```python
from build123d import *

# Parameters (mm, degrees)
SKETCH2_R           = 3.5
BOSS_EXTRUDE1_DEPTH = 1.2
SKETCH3_R           = 0.875
CUT_EXTRUDE1_DEPTH  = 47.574778582
SKETCH10_R          = 2
CUT_EXTRUDE4_DEPTH  = 33.9
SKETCH6_OUTSIDE_W   = 38.142
SKETCH6_OUTSIDE_H   = 38.142
CUT_EXTRUDE2_DEPTH  = 3
FILLET1_R           = 0.2
BOSS_EXTRUDE2_START = 1.5
SKETCH7_W           = 20
SKETCH7_H           = 16
BOSS_EXTRUDE2_DEPTH = 11.5
CHAMFER2_SIZE       = 0.5
SKETCH8_R           = 0.2
CUT_EXTRUDE3_DEPTH  = 67.283482105
SKETCH9_W           = 1.6
SKETCH9_H           = 1.6


with BuildPart() as part:
    # Sketch1 → Revolve1 (revolve)
    with BuildSketch(Plane.XY):
        Polygon((0, 0), (-8, 0), (-8, -3.7), (-6, -3.7), (-6, -9.7), (-8, -9.7), (-8, -12.7), (-4, -12.7), (-4, -14.2), (-8, -14.2), (-8, -15.2), (-4, -15.2), (-4, -16.7), (-11, -16.7), (-11, -17.7), (-3, -17.7), (-3, -19.2), (-11, -19.2), (-11, -20.2), (-3, -20.2), (-3, -21.7), (-11, -21.7), (-11, -22.7), (-3, -22.7), (-3, -24.2), (-11, -24.2), (-11, -25.2), (-3, -25.2), (-3, -26.7), (-11, -26.7), (-11, -27.7), (-3, -27.7), (-3, -29.2), (-11, -29.2), (-11, -30.2), (-3, -30.2), (-3, -31.7), (-11, -31.7), (-11, -32.7), (-3, -32.7), (-3, -34.2), (-11, -34.2), (-11, -35.2), (-3, -35.2), (-3, -36.7), (-11, -36.7), (-11, -37.7), (-3, -37.7), (-3, -39.2), (-11, -39.2), (-11, -40.2), (-3, -40.2), (-3, -41.7), (-11, -41.7), (-11, -42.7), (0, -42.7), align=None)
    revolve(axis=Axis((0, 0, 0), (0, -1, 0)))

    # Sketch2 → Boss-Extrude1 (add)
    with BuildSketch(Plane(origin=(0, 0, 0), x_dir=(1, 0, 0), z_dir=(0, 1, 0))):
        with Locations(Location((0, 0, 0), (0, 0, 180))):
            Circle(SKETCH2_R)
    extrude(amount=BOSS_EXTRUDE1_DEPTH)

    # Sketch3 → Cut-Extrude1 (cut, through all)
    with BuildSketch(Plane(origin=(0, 1.2, 0), x_dir=(1, 0, 0), z_dir=(0, 1, 0))):
        with Locations(Location((0, 0, 0), (0, 0, 180))):
            Circle(SKETCH3_R)
    extrude(amount=-CUT_EXTRUDE1_DEPTH, mode=Mode.SUBTRACT)

    # Sketch10 → Cut-Extrude4 (cut)
    with BuildSketch(Plane(origin=(0, 1.2, 0), x_dir=(1, 0, 0), z_dir=(0, 1, 0))):
        with Locations(Location((0, 0, 0), (0, 0, 180))):
            Circle(SKETCH10_R)
    extrude(amount=-CUT_EXTRUDE4_DEPTH, mode=Mode.SUBTRACT)

    # Sketch5 → Revolve2 (revolve)
    with BuildSketch(Plane.XY, mode=Mode.PRIVATE) as revolve2_sk:
        Polygon((0, -42.7), (-2.5, -42.7), (-2.5, -57.3), (-5, -57.3), (-5, -60.3), (-1.715415076, -60.3), (-0.315, -62.3), (0, -62.3), align=None)
    revolve(revolve2_sk.sketch.rotate(Axis((0, -62.3, 0), (0, 1, 0)), 270), axis=Axis((0, -62.3, 0), (0, 1, 0)))

    # Sketch6 outside → Cut-Extrude2 (cut)
    with BuildSketch(Plane.XZ.offset(60.3)):
        Rectangle(SKETCH6_OUTSIDE_W, SKETCH6_OUTSIDE_H)
        Polygon((2.020725942, 3.5), (-2.020725942, 3.5), (-4.041451884, 0), (-2.020725942, -3.5), (2.020725942, -3.5), (4.041451884, 0), align=None, mode=Mode.SUBTRACT)
    extrude(amount=-CUT_EXTRUDE2_DEPTH, mode=Mode.SUBTRACT)

    # Fillet1
    fillet1_edges = [part.edges().sort_by_distance(p)[0] for p in [
        (2.020725942, -58.8, 3.5),
        (-2.020725942, -58.8, 3.5),
        (-4.041451884, -58.8, 0),
        (-2.020725942, -58.8, -3.5),
        (2.020725942, -58.8, -3.5),
        (4.041451884, -58.8, 0),
    ]]
    fillet(fillet1_edges, radius=FILLET1_R)

    # Sketch7 → Boss-Extrude2 (add)
    with BuildSketch(Plane(origin=(0, -57.3, 0), x_dir=(1, 0, 0), z_dir=(0, 1, 0)).offset(BOSS_EXTRUDE2_START)):
        with Locations((-5.5, 0)):
            Rectangle(SKETCH7_W, SKETCH7_H)
    extrude(amount=BOSS_EXTRUDE2_DEPTH)

    # Chamfer2
    chamfer2_edges = [part.edges().sort_by_distance(p)[0] for p in [
        (4.5, -55.8, 0),
        (4.5, -50.05, 8),
        (-5.5, -55.8, -8),
        (4.5, -50.05, -8),
        (-15.5, -55.8, 0),
        (-15.5, -50.05, -8),
        (-5.5, -55.8, 8),
        (-15.5, -50.05, 8),
        (4.5, -44.3, 0),
        (-5.5, -44.3, -8),
        (-15.5, -44.3, 0),
        (-5.5, -44.3, 8),
    ]]
    chamfer(chamfer2_edges, length=CHAMFER2_SIZE)

    # Sketch8 → Cut-Extrude3 (cut, through all)
    with BuildSketch(Plane.XZ.offset(62.3)):
        with Locations(Location((0, 0, 0), (0, 0, 270))):
            Circle(SKETCH8_R)
    extrude(amount=-CUT_EXTRUDE3_DEPTH, mode=Mode.SUBTRACT)

    # Sketch9 → Cut-Revolve1 (revolve, cut)
    with BuildSketch(Plane.XY, mode=Mode.PRIVATE) as cut_revolve1_sk:
        with Locations((-2.2, -43.5)):
            Rectangle(SKETCH9_W, SKETCH9_H)
    revolve(cut_revolve1_sk.sketch.rotate(Axis((0, -42.7, 0), (0, -1, 0)), 270), axis=Axis((0, -42.7, 0), (0, -1, 0)), mode=Mode.SUBTRACT)


solid = part.part
```
Build history of the part. All positions in model axes, mm. A direction names the side the tool comes from. Round coordinates to 2 decimals unless told otherwise and drop trailing zeros. Loops run counter-clockwise (first coordinate to the right, second up) from the corner with the lowest first, then second, coordinate; pieces in that order, holes last.
Item 1: Pin check, flat tips, straight feed: P1, Ø3, axis at y = -48, z = -3, coming from the +X side; P2, Ø2, axis at x = -7, z = -8.5, coming from the +Y side; P3, Ø6.5, axis at x = 4, z = -1, coming from the -Y side. Stop position of each tip, or through.
Item 2: Which spindle directions (+Z, -Z, +X, -X, +Y, -Y) get a long thin tool onto all of the face, cutting with end or side? Do faces 1 (the face through (0, -59, 3.5)), 2 (the face through (2.38, -29.71, 10.74)), 3 (the face through (3.044, -58.821, 1.727)), 4 (the face through (0, -59, -3.5)). Say none if no direction does.
Item 3: Saw through at A-A (y = -11.5). List the corners of the cut face in (x, z), then the cut area to 3 significant figures.
Item 4: Saw through at B-B (z = -5). State how many separate pieces and enclosed holes the cut face has, then the cut area to 3 significant figures.
Item 5: Drill centre lines: line 1 along Y through (x, z) = (-2.25, 1.25); line 2 along Z through (x, y) = (0, -34.75) (3 decimals); line 3 along Z through (x, y) = (0, -39) (3 decimals). Where is each one in solid material? Low to high.
Worked answers:
1. P1: stops at x = 4.5
1. P2: stops at y = -16.7
1. P3: stops at y = -61.5
2. face 1: +Z, +X, -X, -Y
2. face 2: +Y
2. face 3: +Z, +X, -Y
2. face 4: -Z, +X, -X, -Y
3. outline: circle Ø16 at (0, 0); hole circle Ø4 at (0, 0)
3. area: 188 mm2
4. separate pieces: 14
4. enclosed holes: 0
4. area: 581 mm2
5. line 1: y = -60.3 to -57.3, -55.8 to -44.3, -42.7 to 1.2
5. line 2: z = -11 to -0.875, 0.875 to 11
5. line 3: z = -3 to -0.875, 0.875 to 3
